Geometry check sheet. Reference: the model listing, model coordinates, mm. Round coordinates to 2 decimals unless told otherwise and drop trailing zeros. Order: outer loops, then holes, each group sorted by start corner. A loop starts at its lowest first (then second) coordinate and runs counter-clockwise, first axis right, second up. Notation, with made-up numbers: (26.25, -16.5) - (66.25, -16.5) arc R21 cw to (66.25, -10.5) - close; hole circle Ø3 at (-7.75, 86.25). An arc over 180 degrees is marked (long way). Write each question's results on one line, items separated by ' | '.
```python
from build123d import *

# Parameters (mm, degrees)
SKETCH1_W           = 5
SKETCH1_H           = 35
SKETCH1_R           = 1.625
BOSS_EXTRUDE1_DEPTH = 4
FILLET1_R           = 5


with BuildPart() as part:
    # Sketch1 → Boss-Extrude1 (new body)
    with BuildSketch(Plane.XY):
        Rectangle(SKETCH1_W, SKETCH1_H)
        with Locations((0, -15)):
            Circle(SKETCH1_R, mode=Mode.SUBTRACT)
    extrude(amount=BOSS_EXTRUDE1_DEPTH)

    # Fillet1
    # the kernel refuses this fillet: 5 mm, written as the material it takes off along each edge
    with BuildSketch(Plane(origin=(-2.5, 17.5, -12.5), x_dir=(1, 0, 0), z_dir=(0, 0, 1)), Plane(origin=(2.5, 17.5, -12.5), x_dir=(0, -1, 0), z_dir=(0, 0, 1))) as fillet1_piece_1:
        with BuildLine():
            CenterArc((FILLET1_R, -FILLET1_R), FILLET1_R, 90, 90)
            Line((0, -FILLET1_R), (0, 0))
            Line((0, 0), (FILLET1_R, 0))
        make_face()
    extrude(amount=29, mode=Mode.SUBTRACT)


solid = part.part
```
(1) Section check B-B (z = 0.7). Record the cut outline in (x, y) (3 decimals).
Answers follow:
outline: (-2.5, -17.5) - (2.5, -17.5) - (2.5, 12.5) arc R5 ccw to (0, 16.83) arc R5 ccw to (-2.5, 12.5) - close; hole circle Ø3.25 at (0, -15)
(2) Section check C-C (x = -1). Record the cut outline in (y, z), then the cut area to 3 significant figures.
Answers follow:
outline: (-17.5, 0) - (-16.28, 0) - (-16.28, 4) - (-17.5, 4) - close; (-13.72, 0) - (16.07, 0) - (16.07, 4) - (-13.72, 4) - close | area: 124 mm²
(3) Depth check by flat-ended pin: pin 1 Ø2.5 at (x, y) = (0, -15) entering from +Z. Enter the tip coordinate at first touch or a pass-through.
Answers follow:
pin 1: through
(4) Section check A-A (y = -15). Record the cut outline in (x, z) (3 decimals).
Answers follow:
outline: (-2.5, 0) - (-1.625, 0) - (-1.625, 4) - (-2.5, 4) - close; (1.625, 0) - (2.5, 0) - (2.5, 4) - (1.625, 4) - close
(5) Section check D-D (x = 1.95). Record the cut outline in (y, z).
Answers follow:
outline: (-17.5, 0) - (14.78, 0) - (14.78, 4) - (-17.5, 4) - close
(6) Material ranges on line 1 (Y direction, x = 0.55, z = 0.5); line 2 (Y direction, x = -1.45, z = 2.4); line 3 (Y direction, x = 1.8, z = 2.8), recorded low to high.
Answers follow:
line 1: -17.5 to -16.53, -13.47 to 16.46 | line 2: -17.5 to -15.73, -14.27 to 15.57 | line 3: -17.5 to 15.05
(7) Draft check along X on faces 1 (the face through (0, -17.5, 2)), 2 (the face through (-0.352, -16.586, 1.972)), 3 (the face through (1.848, 14.968, 1.972)), 4 (the face through (-1.812, 15.032, 1.972)). Enter one of: released by +X, released by -X, zero draft, split by the parting line, or undercut.
Answers follow:
face 1: zero draft | face 2: undercut | face 3: released by +X | face 4: released by -X
